```python
from build123d import *

# Parameters (mm, degrees)
F1_DEPTH       = 76.2
F2_R           = 10.16
F4_D           = 15.24
F4_CBORE_D     = 40.64
F4_CBORE_DEPTH = 10.16
F5_R           = 10.16
F6_DEPTH       = 76.201
F8_W           = 10.16
F8_H           = 10.16
F9_DEPTH       = 149.556668
F10_DEPTH      = 71.121


with BuildPart() as f1:
    # F0 (on Right) → F1 (new body)
    with BuildSketch(Plane.YZ):
        Polygon((76.2, 35.56), (0, 35.56), (0, 0), (111.76, 0), (149.555668, 35.56), (149.555668, 71.12), (113.995668, 71.12), align=None)
    extrude(amount=-F1_DEPTH)

    # F2
    f2_edges = [f1.edges().sort_by_distance(p)[0] for p in [
        (-76.2, 0, 17.78),
        (0, 0, 17.78),
    ]]
    fillet(f2_edges, radius=F2_R)

    # F4 (through all)
    with Locations(Plane.XY.offset(35.56)):
        with Locations((-38.1, 38.1)):
            CounterBoreHole(F4_D / 2, F4_CBORE_D / 2, F4_CBORE_DEPTH)

    # F5 (on face) → F6 (cut, through all)
    with BuildSketch(Plane.YZ):
        with Locations((96.215668, 20.32)):
            Circle(F5_R)
    extrude(amount=-F6_DEPTH, mode=Mode.SUBTRACT)

    # F8 (on face) → F9 (cut, through all)
    with BuildSketch(Plane.XZ):
        with Locations((-37.720058, 30.48)):
            Rectangle(F8_W, F8_H)
    extrude(amount=-F9_DEPTH, mode=Mode.SUBTRACT)

    # F7 (on face) → F10 (cut, through all)
    with BuildSketch(Plane.XY.offset(71.12)):
        with BuildLine():
            Line((-15.24, 139.395668), (-60.96, 139.395668))
            ThreePointArc((-60.96, 139.395668), (-68.58, 131.775668), (-60.96, 124.155668))
            Line((-60.96, 124.155668), (-15.24, 124.155668))
            ThreePointArc((-15.24, 124.155668), (-7.62, 131.775668), (-15.24, 139.395668))
        make_face()
    extrude(amount=-F10_DEPTH, mode=Mode.SUBTRACT)


solid = f1.part
```
Input: part model. Units: mm. Frame: model coordinates. A direction names the side the tool comes from. Give positions to 0.01 mm unless a question says otherwise; leave off trailing zeros. Loops run counter-clockwise (first coordinate to the right, second up) from the corner with the lowest first, then second, coordinate; pieces in that order, holes last. Notation, with made-up numbers: (69.5, -12) -> (100.5, -12) arc R14 ccw to (100.5, 11) -> close; hole circle Ø7 at (58, -31). An arc over 180 degrees is marked (long way). Use a Markdown table: item, result.
Q1. Section query A-A, the plane x = -38.1. Return the cut outline in (y, z), plus the area to 3 significant figures.
Entries:
| item | result |
|---|---|
| outline | (0, 0) -> (30.48, 0) -> (30.48, 25.4) -> (0, 25.4) -> close; (45.72, 0) -> (111.76, 0) -> (124.16, 11.66) -> (124.16, 25.4) -> (105.01, 25.4) arc R10.16 cw (long way) to (87.42, 25.4) -> (45.72, 25.4) -> close; (76.2, 35.56) -> (124.16, 35.56) -> (124.16, 71.12) -> (114, 71.12) -> close; (139.4, 35.56) -> (149.56, 35.56) -> (149.56, 71.12) -> (139.4, 71.12) -> close |
| area | 3,830 mm² |
Q2. Section query D-D, the plane x = -63.5. Return the cut outline in (y, z), plus the area to 3 significant figures.
Entries:
| item | result |
|---|---|
| outline | (0, 0) -> (111.76, 0) -> (124.59, 12.07) -> (124.59, 71.12) -> (114, 71.12) -> (76.2, 35.56) -> (0, 35.56) -> close; (138.96, 25.59) -> (149.56, 35.56) -> (149.56, 71.12) -> (138.96, 71.12) -> close; hole circle Ø20.32 at (96.22, 20.32) |
| area | 5,510 mm² |
Q3. Section query B-B, the plane y = 38.1. Return the cut outline in (x, z).
Entries:
| item | result |
|---|---|
| outline | (-76.2, 0) -> (-45.72, 0) -> (-45.72, 25.4) -> (-58.42, 25.4) -> (-58.42, 35.56) -> (-76.2, 35.56) -> close; (-30.48, 0) -> (0, 0) -> (0, 35.56) -> (-17.78, 35.56) -> (-17.78, 25.4) -> (-30.48, 25.4) -> close |
Q4. First-contact query: P1, Ø10, axis at y = 41, z = 45, coming from the -X side; P2, Ø10, axis at x = -34.5, y = 75, coming from the +Z side; P3, Ø3, axis at x = -49.5, z = 52.5, coming from the -Y side; P4, Ø8, axis at x = -37.5, y = 105, coming from the -Z side. Flat tips, straight axial feed; report the tip coordinate or a pass-through.
Entries:
| item | result |
|---|---|
| P1 | passes through |
| P2 | stops at z = 39.14 |
| P3 | stops at y = 92.61 |
| P4 | stops at z = 0 |
Q5. Section query C-C, the plane z = 14. Return the cut outline in (x, y).
Entries:
| item | result |
|---|---|
| outline | (-76.2, 10.16) arc R10.16 ccw to (-66.04, 0) -> (-10.16, 0) arc R10.16 ccw to (0, 10.16) -> (0, 88.26) -> (-76.2, 88.26) -> close; (-76.2, 104.17) -> (0, 104.17) -> (0, 126.64) -> (-9.61, 126.64) arc R7.62 cw to (-15.24, 124.16) -> (-60.96, 124.16) arc R7.62 cw to (-66.59, 126.64) -> (-76.2, 126.64) -> close; hole circle Ø15.24 at (-38.1, 38.1) |
Q6. Ray query, probe 1 along Y at (x, z) = (-44, 28); probe 2 along X at (y, z) = (38, 14); probe 3 along Y at (x, z) = (-38, 17). Return the intervals inside material, ascending. Write a range as from..to.
Entries:
| item | result |
|---|---|
| probe 1 | y = 0..18.66, 57.54..89.56, 102.87..124.16, 139.4..141.52 |
| probe 2 | x = -76.2..-45.72, -30.48..0 |
| probe 3 | y = 0..30.48, 45.72..86.61, 105.82..124.16 |
Q7. Access query for faces 4 (the flat face through (-38, 139.396, 49)), 5 (the flat face through (-42.8, 91, 30)), 6 (the flat face through (-42.8, 142, 33)), 7 (the flat face through (-42.8, 9, 30)). Directions: +Z, -Z, +X, -X, +Y, -Y. A direction counts if a zero-diameter tool reaches every point of the face in a straight line with its end or side. Return the directions, or none.
Entries:
| item | result |
|---|---|
| face 4 | +Z, -Z |
| face 5 | +Y, -Y |
| face 6 | -Z, +Y, -Y |
| face 7 | +Z, +Y, -Y |
Q8. Pull-direction query (Z, two-part tool) for faces 1 (the flat face through (-38, 100, 35.56)), 2 (the cylindrical face through (-73.145, 2.897, 17.531)), 3 (the flat face through (-38, 144, 35.56)); classes: pulls with the +Z half, pulls with the -Z half, needs draft (parallel to the pull), parting line crosses it, or undercut.
Entries:
| item | result |
|---|---|
| face 1 | undercut |
| face 2 | needs draft |
| face 3 | pulls with the -Z half |
